```python
from build123d import *

# Parameters (mm, degrees)
SKETCH1_W           = 190.5
SKETCH1_H           = 190.5
BOSS_EXTRUDE1_DEPTH = 9.525
SKETCH4_R           = 3.1242
CUT_EXTRUDE1_DEPTH  = 270.576010849
CUT_EXTRUDE2_DEPTH  = 2.032
CUT_EXTRUDE3_DEPTH  = 6.35
SKETCH7_R           = 3.175
CUT_EXTRUDE4_DEPTH  = 1.524
LPATTERN1_COUNT     = 4
LPATTERN1_PITCH     = 44.45
LPATTERN2_COUNT     = 4
LPATTERN2_PITCH     = 44.45
SKETCH8_R           = 4.7625
CUT_EXTRUDE5_DEPTH  = 270.576010849
FILLET1_R           = 6.35


with BuildPart() as part:
    # Sketch1 → Boss-Extrude1 (new body)
    with BuildSketch(Plane.XY):
        with Locations((95.25, 95.25)):
            Rectangle(SKETCH1_W, SKETCH1_H)
    extrude(amount=BOSS_EXTRUDE1_DEPTH)

    # Sketch4 → Cut-Extrude1 (cut, through all)
    with BuildSketch(Plane.XY.offset(9.525)):
        with Locations((6.35, 6.35)):
            Circle(SKETCH4_R)
        with Locations((6.35, 184.15)):
            Circle(SKETCH4_R)
        with Locations((184.15, 184.15)):
            Circle(SKETCH4_R)
        with Locations((184.15, 6.35)):
            Circle(SKETCH4_R)
    cut_extrude1 = extrude(amount=-CUT_EXTRUDE1_DEPTH, mode=Mode.SUBTRACT)

    # Sketch5 → Cut-Extrude2 (cut)
    with BuildSketch(Plane.XY.offset(9.525)):
        with BuildLine():
            Line((19.05, 177.8), (171.45, 177.8))
            ThreePointArc((171.45, 177.8), (175.940128061, 175.940128061), (177.8, 171.45))
            Line((177.8, 171.45), (177.8, 19.05))
            ThreePointArc((177.8, 19.05), (175.940128061, 14.559871939), (171.45, 12.7))
            Line((171.45, 12.7), (19.05, 12.7))
            ThreePointArc((19.05, 12.7), (14.559871939, 14.559871939), (12.7, 19.05))
            Line((12.7, 19.05), (12.7, 171.45))
            ThreePointArc((12.7, 171.45), (14.559871939, 175.940128061), (19.05, 177.8))
        make_face()
        with BuildLine():
            ThreePointArc((171.45, 14.2875), (174.817596045, 15.682403955), (176.2125, 19.05))
            Line((176.2125, 19.05), (176.2125, 171.45))
            ThreePointArc((176.2125, 171.45), (174.817596045, 174.817596045), (171.45, 176.2125))
            Line((171.45, 176.2125), (19.05, 176.2125))
            ThreePointArc((19.05, 176.2125), (15.682403955, 174.817596045), (14.2875, 171.45))
            Line((14.2875, 171.45), (14.2875, 19.05))
            ThreePointArc((14.2875, 19.05), (15.682403955, 15.682403955), (19.05, 14.2875))
            Line((19.05, 14.2875), (171.45, 14.2875))
        make_face(mode=Mode.SUBTRACT)
    extrude(amount=-CUT_EXTRUDE2_DEPTH, mode=Mode.SUBTRACT)

    # Sketch6 → Cut-Extrude3 (cut)
    with BuildSketch(Plane.XY.offset(9.525)):
        with BuildLine():
            Line((173.0375, 19.05), (173.0375, 171.45))
            ThreePointArc((173.0375, 171.45), (172.572532015, 172.572532015), (171.45, 173.0375))
            Line((171.45, 173.0375), (19.05, 173.0375))
            ThreePointArc((19.05, 173.0375), (17.927467985, 172.572532015), (17.4625, 171.45))
            Line((17.4625, 171.45), (17.4625, 19.05))
            ThreePointArc((17.4625, 19.05), (17.927467985, 17.927467985), (19.05, 17.4625))
            Line((19.05, 17.4625), (171.45, 17.4625))
            ThreePointArc((171.45, 17.4625), (172.572532015, 17.927467985), (173.0375, 19.05))
        make_face()
    extrude(amount=-CUT_EXTRUDE3_DEPTH, mode=Mode.SUBTRACT)

    # Sketch7 → Cut-Extrude4 (cut)
    with BuildSketch(Plane.XY.offset(3.175)):
        with Locations((22.225, 168.275)):
            Circle(SKETCH7_R)
        with Locations((168.275, 168.275)):
            Circle(SKETCH7_R)
        with Locations((22.225, 22.225)):
            Circle(SKETCH7_R)
        with Locations((168.275, 22.225)):
            Circle(SKETCH7_R)
        with Locations((95.25, 168.275)):
            Circle(SKETCH7_R)
        with Locations((22.225, 95.25)):
            Circle(SKETCH7_R)
        with Locations((168.275, 95.25)):
            Circle(SKETCH7_R)
        with Locations((95.25, 22.225)):
            Circle(SKETCH7_R)
    extrude(amount=-CUT_EXTRUDE4_DEPTH, mode=Mode.SUBTRACT)

    # LPattern1: Cut-Extrude1 ×4
    with Locations(*[(0, -i * LPATTERN1_PITCH, 0) for i in range(1, LPATTERN1_COUNT)]):
        add(cut_extrude1, mode=Mode.SUBTRACT)

    # LPattern2: Cut-Extrude1 ×4
    with Locations(*[(i * LPATTERN2_PITCH, 0, 0) for i in range(1, LPATTERN2_COUNT)]):
        add(cut_extrude1, mode=Mode.SUBTRACT)

    # Sketch8 → Cut-Extrude5 (cut, through all)
    with BuildSketch(Plane.XY.offset(9.525)):
        with Locations((95.25, 184.15)):
            Circle(SKETCH8_R)
        with Locations((95.25, 6.35)):
            Circle(SKETCH8_R)
    extrude(amount=-CUT_EXTRUDE5_DEPTH, mode=Mode.SUBTRACT)

    # Fillet1
    fillet1_edges = [part.edges().sort_by_distance(p)[0] for p in [
        (0, 190.5, 4.7625),
        (190.5, 190.5, 4.7625),
        (190.5, 0, 4.7625),
        (0, 0, 4.7625),
    ]]
    fillet(fillet1_edges, radius=FILLET1_R)


solid = part.part
```
Design review of the part built by this model. Coordinates are the model's own, in mm. A direction names the side the tool comes from. Give positions to 0.01 mm unless a question says otherwise; leave off trailing zeros. Order: outer loops, then holes, each group sorted by start corner. A loop starts at its lowest first (then second) coordinate and runs counter-clockwise, first axis right, second up. Notation, with made-up numbers: (-3, 38.25) -> (10, 38.25) arc R24 ccw to (10, 57.25) -> close; hole circle Ø10 at (39.5, -13.75). An arc over 180 degrees is marked (long way). Write each question's results on one line, items separated by ' | '. Start each with the question number.
Q1. Machinability: for faces 1 (the cylindrical face through (90.492, 184.359, 4.829)), 2 (the flat face through (168, 168, 1.651)), which of the approach directions +Z, -Z, +X, -X, +Y, -Y give a long, thin tool a straight path to every point of the face, cutting with its end or side? Answer none if there is none.
Q2. For pin 1 (5 mm diameter, centred on x = 26.5, y = 120.5, fed in from +Z) (3 decimals); pin 2 (3 mm diameter, centred on x = 167.5, y = 23, fed in from +Z), all flat-tipped, find the tip position at first contact; note any pin that passes through.
Q3. Mouldability with a two-part tool opening along X and no side actions: class faces 3 (the cylindrical face through (185.83, 97.884, 4.829)), 4 (the flat face through (0, 94, 5)), 5 (the flat face through (10, 96, 9.525)) as +X half, -X half, draft (parallel to the pull), parting line (faces both ways), or undercut.
Q4. Add section A-A on x = 95.25. State how many separate pieces and enclosed holes the cut face has, and give its area (3 significant figures).
Q5. Add section C-C on x = 64. Give the boundary of the cut face in (y, z) (1 decimal).
Q6. Wall thickness on L1, parallel to Y at x = 184.15, z = 4; L2, parallel to X at y = 125, z = 7.75; L3, parallel to Y at x = 139.7, z = 3.25: over which ranges is each line inside the solid? List them lowest first. Write a range as from..to.
Found:
1) face 1: +Z, -Z | face 2: +Z
2) pin 1: stops at z = 3.175 | pin 2: stops at z = 1.65
3) face 3: undercut | face 4: -X half | face 5: draft
4) separate pieces: 3 | enclosed holes: 0 | area: 619 mm2
5) outline: (0, 0) -> (190.5, 0) -> (190.5, 9.5) -> (177.8, 9.5) -> (177.8, 7.5) -> (176.2, 7.5) -> (176.2, 9.5) -> (173, 9.5) -> (173, 3.2) -> (17.5, 3.2) -> (17.5, 9.5) -> (14.3, 9.5) -> (14.3, 7.5) -> (12.7, 7.5) -> (12.7, 9.5) -> (0, 9.5) -> close
6) L1: y = 0..3.23, 9.47..47.68, 53.92..92.13, 98.37..136.58, 142.82..181.03, 187.27..190.5 | L2: x = 0..12.7, 14.29..17.46, 173.04..176.21, 177.8..190.5 | L3: y = 0..3.23, 9.47..17.46, 173.04..181.03, 187.27..190.5
